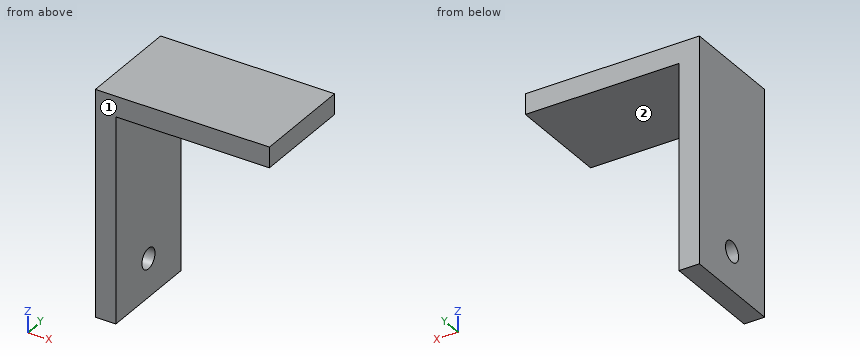
```python
from build123d import *

# Parameters (mm, degrees)
F0_W     = 38.1
F0_H     = 5.08
F1_DEPTH = 25.4
F2_R     = 2.54
F3_DEPTH = 25.4


with BuildPart() as f1:
    # F0 (on Front) → F1 (new body)
    with BuildSketch(Plane.XZ):
        with Locations((24.13, 53.34)):
            Rectangle(F0_W, F0_H)
        Polygon((0, 55.88), (0, 0), (5.08, 0), (5.08, 50.8), (5.08, 55.88), align=None)
    extrude(amount=F1_DEPTH)

    # F2 (on face) → F3 (cut)
    with BuildSketch(Plane(origin=(0, 0, 0), x_dir=(0, -1, 0), z_dir=(-1, 0, 0))):
        with Locations((12.7, 9.525)):
            Circle(F2_R)
    extrude(amount=-F3_DEPTH, mode=Mode.SUBTRACT)


solid = f1.part
```
The model under review builds one solid part; all positions refer to its coordinate system, in mm. Face numbers are marked on the shaded views. A direction names the side the tool comes from. Round coordinates to 2 decimals unless told otherwise and drop trailing zeros. Order: outer loops, then holes, each group sorted by start corner. A loop starts at its lowest first (then second) coordinate and runs counter-clockwise, first axis right, second up. Notation, with made-up numbers: (69, -37) -> (78, -37) arc R25 cw to (78, 1) -> close; hole circle Ø8 at (61, 38.25). An arc over 180 degrees is marked (long way). Use a Markdown table: item, result.
Q1. We need section B-B on x = 10. Write out the cut boundary in (y, z).
Values:
| item | result |
|---|---|
| outline | (-25.4, 50.8) -> (0, 50.8) -> (0, 55.88) -> (-25.4, 55.88) -> close |
Q2. For line 1 (Z direction, x = 3.9, y = -12.7) (3 decimals); line 2 (X direction, y = -6.75, z = 41.5); line 3 (Z direction, x = 17, y = -12), list the stretches that pass through material, from the lowest coordinate up.
Values:
| item | result |
|---|---|
| line 1 | z = 0 to 6.985, 12.065 to 55.88 |
| line 2 | x = 0 to 5.08 |
| line 3 | z = 50.8 to 55.88 |
Q3. We need section C-C on y = -3.75. Write out the cut boundary in (x, z).
Values:
| item | result |
|---|---|
| outline | (0, 0) -> (5.08, 0) -> (5.08, 50.8) -> (43.18, 50.8) -> (43.18, 55.88) -> (0, 55.88) -> close |
Q4. Tool access review of the marked faces 1 and 2: name each direction out of +Z, -Z, +X, -X, +Y, -Y from which nothing blocks a thin tool from reaching the whole face with its end or side.
Values:
| item | result |
|---|---|
| face 1 | +Z, -Z, +X, -X, -Y |
| face 2 | -Z, +X, +Y, -Y |
Q5. We need section D-D on z = 33. Write out the cut boundary in (x, y), then the cut area to 3 significant figures.
Values:
| item | result |
|---|---|
| outline | (0, -25.4) -> (5.08, -25.4) -> (5.08, 0) -> (0, 0) -> close |
| area | 129 mm^2 |
Q6. Clearance check with flat-ended pins moving along their axes: P1, Ø8, axis at y = -17.5, z = 27, coming from the -X side; P2, Ø12, axis at y = -17.5, z = 34.5, coming from the +X side; P3, Ø8, axis at x = 17.5, y = -12, coming from the -Z side. State where each tip first meets the part, or that it passes through.
Values:
| item | result |
|---|---|
| P1 | stops at x = 0 |
| P2 | stops at x = 5.08 |
| P3 | stops at z = 50.8 |
Q7. We need section A-A on y = -12.7. Write out the cut boundary in (x, z) (3 decimals), then the cut area to 3 significant figures.
Values:
| item | result |
|---|---|
| outline | (0, 0) -> (5.08, 0) -> (5.08, 6.985) -> (0, 6.985) -> close; (0, 12.065) -> (5.08, 12.065) -> (5.08, 50.8) -> (43.18, 50.8) -> (43.18, 55.88) -> (0, 55.88) -> close |
| area | 452 mm^2 |
